Build history of the part. All positions in model axes, mm. A direction names the side the tool comes from. Round coordinates to 2 decimals unless told otherwise and drop trailing zeros. Write each loop counter-clockwise with the first axis right and the second up, starting at its lowest first coordinate (ties: lowest second). Pieces come first, ordered by that corner, then holes.
Item 1: 3-axis set-ups, long thin cutter, end or side, ignore diameter. For faces 1 (the flat face through (-4, 0, -3)), 2 (the cylindrical face through (-2.85, 2.99, -5.28)): which of +Z, -Z, +X, -X, +Y, -Y reach the whole face in a straight line?
Item 2: Band-saw the part on C-C, the plane y = 1.25. Write the cut outline in (x, z), then the cut area to 3 significant figures.
Item 3: Drop a flat-ended pin along its axis: pin 1 Ø3 at (x, z) = (6.5, -12) entering from +Y. Give the stop position or say it passes through.
Item 4: Band-saw the part on D-D, the plane y = 4. Write the cut outline in (x, z).
Item 5: Mould opens along Z. For faces 3 (the flat face through (-4, 5, 4)), 4 (the cylindrical face through (0.66, 1.232, -14.985)), 5 (the cylindrical face through (-1.519, 2.993, 7.345)) say: +Z half, -Z half, draft (parallel to the pull), parting line (faces both ways), or undercut.
Item 6: Wall check: probe 1 along X at (y, z) = (1.4, 0); probe 2 along X at (y, z) = (1, -4.75); probe 3 along Y at (x, z) = (-8.25, 0.5). Give the ranges that are in metal, low to high.
```python
from build123d import *

# Parameters (mm, degrees)
SKETCH1_R           = 15
BOSS_EXTRUDE1_DEPTH = 5
SKETCH2_R           = 8.6
CUT_EXTRUDE1_DEPTH  = 2.5
SKETCH5_R           = 4.65
CUT_EXTRUDE2_DEPTH  = 2.5
CUT_EXTRUDE3_DEPTH  = 1
SKETCH7_R           = 6
SKETCH7_R_2         = 4.65
BOSS_EXTRUDE2_DEPTH = 2.5


with BuildPart() as part:
    # Sketch1 → Boss-Extrude1 (new body)
    with BuildSketch(Plane(origin=(0, 0, 0), x_dir=(1, 0, 0), z_dir=(0, 1, 0))):
        with Locations(Location((0, 0, 0), (0, 0, 270))):
            Circle(SKETCH1_R)
    extrude(amount=BOSS_EXTRUDE1_DEPTH)

    # Sketch2 → Cut-Extrude1 (cut)
    with BuildSketch(Plane.XZ):
        with Locations(Location((0, 0, 0), (0, 0, 270))):
            Circle(SKETCH2_R)
    extrude(amount=-CUT_EXTRUDE1_DEPTH, mode=Mode.SUBTRACT)

    # Sketch4 → Cut-Revolve1 (revolve, cut)
    with BuildSketch(Plane.XY, mode=Mode.PRIVATE) as cut_revolve1_sk:
        Polygon((8.6, 5), (15, 5), (15, 2.5), align=None)
    revolve(cut_revolve1_sk.sketch.rotate(Axis((0, 2.5, 0), (0, 1, 0)), 90), axis=Axis((0, 2.5, 0), (0, 1, 0)), mode=Mode.SUBTRACT)

    # Sketch5 → Cut-Extrude2 (cut)
    with BuildSketch(Plane(origin=(0, 5, 0), x_dir=(1, 0, 0), z_dir=(0, 1, 0))):
        with Locations(Location((0, 0, 0), (0, 0, 270))):
            Circle(SKETCH5_R)
    extrude(amount=-CUT_EXTRUDE2_DEPTH, mode=Mode.SUBTRACT)

    # Sketch6 → Cut-Extrude3 (cut)
    with BuildSketch(Plane.XZ.offset(-2.5)):
        with BuildLine():
            ThreePointArc((-0.757021, -7.461697), (7.461697, -0.757021), (0.757021, 7.461697))
            ThreePointArc((0.757021, 7.461697), (-7.461697, 0.757021), (-0.757021, -7.461697))
        make_face()
        with BuildLine():
            ThreePointArc((0.605617, 5.969357), (-5.969357, 0.605617), (-0.605617, -5.969357))
            ThreePointArc((-0.605617, -5.969357), (5.969357, -0.605617), (0.605617, 5.969357))
        make_face(mode=Mode.SUBTRACT)
    extrude(amount=-CUT_EXTRUDE3_DEPTH, mode=Mode.SUBTRACT)

    # Sketch7 → Boss-Extrude2 (add)
    with BuildSketch(Plane.XZ.offset(-2.5)):
        with Locations(Location((0, 0, 0), (0, 0, 270))):
            Circle(SKETCH7_R)
        with Locations(Location((0, 0, 0), (0, 0, 90))):
            Circle(SKETCH7_R_2, mode=Mode.SUBTRACT)
    extrude(amount=BOSS_EXTRUDE2_DEPTH)


solid = part.part
```
Results:
1. face 1: +Z, -Z, +X, -X, -Y
1. face 2: -Y
2. outline: circle Ø30 at (0, 0); circle Ø12 at (0, 0); hole circle Ø17.2 at (0, 0); hole circle Ø9.3 at (0, 0)
2. area: 520 mm2
3. pin 1: stops at y = 3.61
4. outline: circle Ø22.32 at (0, 0); hole circle Ø9.3 at (0, 0)
5. face 3: draft
5. face 4: parting line
5. face 5: undercut
6. probe 1: x = -15 to -8.6, -6 to -4.65, 4.65 to 6, 8.6 to 15
6. probe 2: x = -14.23 to -7.17, -3.67 to 3.67, 7.17 to 14.23
6. probe 3: y = 2.5 to 5
